The model under review builds one solid part; all positions refer to its coordinate system, in mm. Face numbers are marked on the shaded views. Give positions to 0.01 mm unless a question says otherwise; leave off trailing zeros. Loops run counter-clockwise (first coordinate to the right, second up) from the corner with the lowest first, then second, coordinate; pieces in that order, holes last. Notation, with made-up numbers: (-8.5, -26.5) - (25.5, -26.5) arc R15 cw to (25.5, -19.5) - close; hole circle Ø9 at (26.5, -36.5). An arc over 180 degrees is marked (long way). Answer as a JSON object with one key per item and string values.
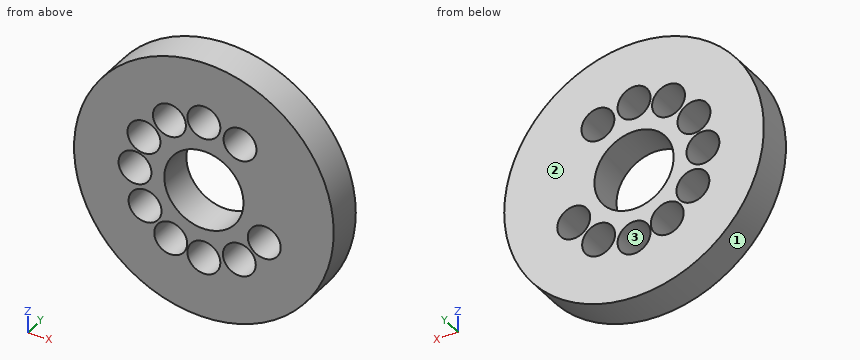
from build123d import *

# Parameters (mm, degrees)
F0_R     = 106.5
F0_R_2   = 75
F0_R_3   = 13.5
F0_R_4   = 37.5
F0_R_5   = 32.5
F1_DEPTH = 30


with BuildPart() as f1:
    # F0 (on Front) → F1 (new body)
    with BuildSketch(Plane.XZ):
        Circle(F0_R)
        Circle(F0_R_2, mode=Mode.SUBTRACT)
        Circle(F0_R_2)
        with Locations((-27.2225671893, -49.5094115863)):
            Circle(F0_R_3, mode=Mode.SUBTRACT)
        with Locations((-48.2611707722, -29.3787235205)):
            Circle(F0_R_3, mode=Mode.SUBTRACT)
        with Locations((0, -56.5)):
            Circle(F0_R_3, mode=Mode.SUBTRACT)
        with Locations((29.0680028111, -48.4489547108)):
            Circle(F0_R_3, mode=Mode.SUBTRACT)
        with Locations((49.5080817216, -27.2249856611)):
            Circle(F0_R_3, mode=Mode.SUBTRACT)
        with Locations((-56.5, 0)):
            Circle(F0_R_3, mode=Mode.SUBTRACT)
        with Locations((-49.1456532959, 27.8739082678)):
            Circle(F0_R_3, mode=Mode.SUBTRACT)
        with Locations((-28.2644325552, 48.9220998357)):
            Circle(F0_R_3, mode=Mode.SUBTRACT)
        Circle(F0_R_4, mode=Mode.SUBTRACT)
        with Locations((29.631335914, 48.1064853419)):
            Circle(F0_R_3, mode=Mode.SUBTRACT)
        with Locations((0, 56.5)):
            Circle(F0_R_3, mode=Mode.SUBTRACT)
        Circle(F0_R_4)
        Circle(F0_R_5, mode=Mode.SUBTRACT)
    extrude(amount=F1_DEPTH)


solid = f1.part
Q1. To check wall thickness, follow probe 1 along Z at (x, y) = (-53, -10.5); probe 2 along Z at (x, y) = (-26, -12); probe 3 along X at (y, z) = (-18.25, 55). State the ranges of each line that lie inside material, in increasing order. Write a range as [from, to].
Results:
{"probe 1": "z = [-92.38, -42.02], [-16.74, -13.04], [13.04, 14.94], [40.81, 92.38]", "probe 2": "z = [-103.28, -62.95], [-36.06, -19.5], [19.5, 35.61], [62.23, 103.28]", "probe 3": "x = [-91.2, -40.32], [-16.21, -13.42], [13.42, 18.02], [41.24, 91.2]"}
Q2. Consider section A-A, the plane x = 0. State the section outline as (y, z) points.
Results:
{"outline": "(-30, -106.5) - (0, -106.5) - (0, -70) - (-30, -70) - close; (-30, -43) - (0, -43) - (0, -32.5) - (-30, -32.5) - close; (-30, 32.5) - (0, 32.5) - (0, 43) - (-30, 43) - close; (-30, 70) - (0, 70) - (0, 106.5) - (-30, 106.5) - close"}
Q3. Clearance check with flat-ended pins moving along their axes: pin 1 Ø3 at (y, z) = (-23.5, -43.5) entering from -X; pin 2 Ø2 at (x, z) = (31, -69) entering from +Y; pin 3 Ø4 at (x, y) = (-21, -13.5) entering from -Z; pin 4 Ø6 at (y, z) = (-13.5, 84) entering from +X. State where each tip first meets the part, or that it passes through.
Results:
{"pin 1": "stops at x = -97.87", "pin 2": "stops at y = 0", "pin 3": "stops at z = -104.79", "pin 4": "stops at x = 69.15"}
Q4. Consider section C-C, the plane z = 56.5. State the section outline as (x, y) points, plus the area to 3 significant figures.
Results:
{"outline": "(-90.28, -30) - (-39.44, -30) - (-39.44, 0) - (-90.28, 0) - close; (-17.09, -30) - (-13.5, -30) - (-13.5, 0) - (-17.09, 0) - close; (13.5, -30) - (19.06, -30) - (19.06, 0) - (13.5, 0) - close; (40.2, -30) - (90.28, -30) - (90.28, 0) - (40.2, 0) - close", "area": "3,300 mm^2"}
Q5. The part is to be moulded in two halves that separate along X. For the marked faces 1, 2 and 3, say which applies: +X half, -X half, draft (parallel to the pull), parting line (faces both ways), or undercut.
Results:
{"face 1": "parting line", "face 2": "draft", "face 3": "undercut"}
Q6. Consider section D-D, the plane y = -13.75. State how many separate pieces and enclosed holes the cut face has, plus the area to 3 significant figures.
Results:
{"separate pieces": "1", "enclosed holes": "11", "area": "26,600 mm^2"}
Q7. Consider section B-B, the plane z = 0. State the section outline as (x, y) points, plus the area to 3 significant figures.
Results:
{"outline": "(-106.5, -30) - (-70, -30) - (-70, 0) - (-106.5, 0) - close; (-43, -30) - (-32.5, -30) - (-32.5, 0) - (-43, 0) - close; (32.5, -30) - (106.5, -30) - (106.5, 0) - (32.5, 0) - close", "area": "3,630 mm^2"}
